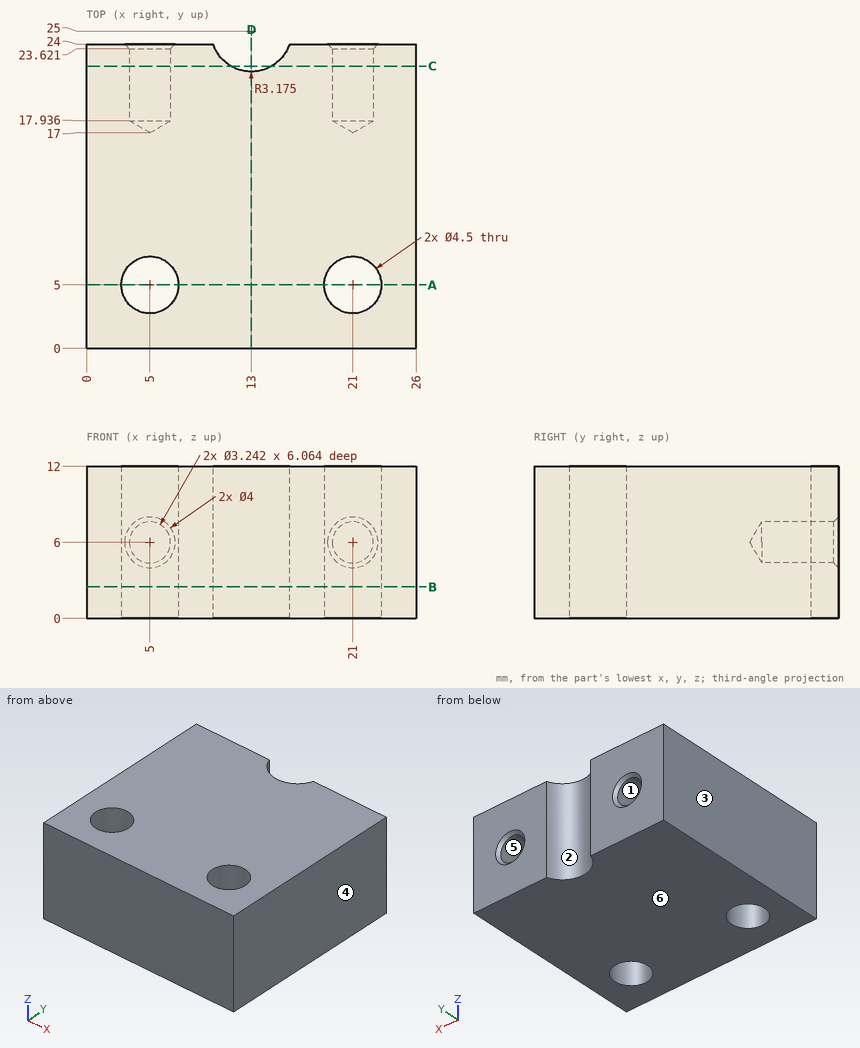
Answer from the drawing. Dimensions are ordinates in mm from the lowest x, y and z of the part. A direction names the side the tool comes from. Round coordinates to 2 decimals unless told otherwise and drop trailing zeros. Order: outer loops, then holes, each group sorted by start corner. A loop starts at its lowest first (then second) coordinate and runs counter-clockwise, first axis right, second up. Notation, with made-up numbers: (8.5, 43) -> (21.5, 43) arc R33 cw to (21.5, 79) -> close; hole circle Ø10 at (13, 28.5). An arc over 180 degrees is marked (long way). Answer as CSV lines item,"result".
Q1. Consider line 1 (X direction, y = 20.35, z = 6); line 2 (Z direction, x = 21, y = 19.4); line 3 (X direction, y = 6, z = 5). Determine where each line is inside the solid, lowest interval first. Write a range as from..to.
Computed values:
line 1,"x = 0..3.38, 6.62..19.38, 22.62..26"
line 2,"z = 0..4.38, 7.62..12"
line 3,"x = 0..2.98, 7.02..18.98, 23.02..26"
Q2. A cutting plane is placed at B-B on z = 2.5. Give the number of separate pieces and of enclosed holes in the cut face, plus the area to 3 significant figures.
Computed values:
separate pieces,"1"
enclosed holes,"2"
area,"583 mm^2"
Q3. For a pull along X with two mould halves and no side action, classify the marked faces 3, 4, 5 and 6 as +X half, -X half, draft (parallel to the pull), parting line (faces both ways), or undercut.
Computed values:
face 3,"-X half"
face 4,"+X half"
face 5,"undercut"
face 6,"draft"
Q4. A cutting plane is placed at A-A on y = 5. Determine the outline of the cut face in (x, z).
Computed values:
outline,"(0, 0) -> (2.75, 0) -> (2.75, 12) -> (0, 12) -> close; (7.25, 0) -> (18.75, 0) -> (18.75, 12) -> (7.25, 12) -> close; (23.25, 0) -> (26, 0) -> (26, 12) -> (23.25, 12) -> close"
Q5. Which of the six approach directions +Z, -Z, +X, -X, +Y, -Y give full straight-line access (tool end or side, diameter ignored) to the marked faces 1 and 2?
Computed values:
face 1,"+Y"
face 2,"+Z, -Z, +Y"
Q6. A cutting plane is placed at C-C on y = 22.25. Determine the outline of the cut face in (x, z).
Computed values:
outline,"(0, 0) -> (11.41, 0) -> (11.41, 12) -> (0, 12) -> close; (14.59, 0) -> (26, 0) -> (26, 12) -> (14.59, 12) -> close; hole circle Ø3.24 at (5, 6); hole circle Ø3.24 at (21, 6)"
Q7. A cutting plane is placed at D-D on x = 13. Determine the outline of the cut face in (y, z) (3 decimals).
Computed values:
outline,"(0, 0) -> (21.825, 0) -> (21.825, 12) -> (0, 12) -> close"
Q8. Given pin 1 (3.5 mm diameter, centred on x = 5, z = 6, fed in from +Y); pin 2 (2.5 mm diameter, centred on x = 21, y = 5, fed in from +Z), each flat-ended and moving along its own axis, determine where each tip first touches the part or whether it passes through.
Computed values:
pin 1,"stops at y = 23.75"
pin 2,"passes through"
